```python
from build123d import *

# Parameters (mm, degrees)
F0_W     = 714.375
F0_H     = 603.123
F1_DEPTH = 3.175
F2_W     = 720.725
F2_H     = 609.473
F2_W_2   = 714.375
F2_H_2   = 603.123
F3_DEPTH = 28.575


with BuildPart() as f1:
    # F0 (on Top) → F1 (new body)
    with BuildSketch(Plane.XY):
        Rectangle(F0_W, F0_H)
    extrude(amount=F1_DEPTH)

    # F2 (on face) → F3 (join)
    with BuildSketch(Plane.XY.offset(3.175)):
        Rectangle(F2_W, F2_H)
        Rectangle(F2_W_2, F2_H_2, mode=Mode.SUBTRACT)
    extrude(amount=-F3_DEPTH)


solid = f1.part
```
Work out the finished part from the listing and answer in its coordinate system (mm). A direction names the side the tool comes from. Round coordinates to 2 decimals unless told otherwise and drop trailing zeros. Write each loop counter-clockwise with the first axis right and the second up, starting at its lowest first coordinate (ties: lowest second). Pieces come first, ordered by that corner, then holes.
1) A cutting plane is placed at A-A on z = -19.5. Determine the outline of the cut face in (x, y), and give its area (3 significant figures).
2) Consider probe 1 along X at (y, z) = (179.5, -22.25); probe 2 along Y at (x, z) = (149, -4); probe 3 along Z at (x, y) = (-126, -265.5) (3 decimals). Determine where each line is inside the solid, lowest interval first.
3) Which of the six approach directions +Z, -Z, +X, -X, +Y, -Y give full straight-line access (tool end or side, diameter ignored) to faces 1 (the face through (-5, -301.562, -13)), 2 (the face through (-5, -304.736, -11))?
4) Determine the mould class of faces 3 (the face through (360.362, -4, -11)), 4 (the face through (357.188, -4, -13)), 5 (the face through (-360.362, -4, -11)) for opening direction X: pulls with the +X half, pulls with the -X half, needs draft (parallel to the pull), parting line crosses it, or undercut.
5) A cutting plane is placed at B-B on x = 34.5. Determine the outline of the cut face in (y, z) (1 decimal).
6) A cutting plane is placed at C-C on y = -72. Determine the outline of the cut face in (x, z) (1 decimal), and give its area (3 significant figures).
Entries:
1. outline: (-360.36, -304.74) - (360.36, -304.74) - (360.36, 304.74) - (-360.36, 304.74) - close; hole (-357.19, -301.56) - (357.19, -301.56) - (357.19, 301.56) - (-357.19, 301.56) - close
1. area: 8,410 mm2
2. probe 1: x = -360.36 to -357.19, 357.19 to 360.36
2. probe 2: y = -304.74 to -301.56, 301.56 to 304.74
2. probe 3: z = 0 to 3.175
3. face 1: -Z
3. face 2: +Z, -Z, +X, -X, -Y
4. face 3: pulls with the +X half
4. face 4: undercut
4. face 5: pulls with the -X half
5. outline: (-304.7, -25.4) - (-301.6, -25.4) - (-301.6, 0) - (301.6, 0) - (301.6, -25.4) - (304.7, -25.4) - (304.7, 3.2) - (-304.7, 3.2) - close
6. outline: (-360.4, -25.4) - (-357.2, -25.4) - (-357.2, 0) - (357.2, 0) - (357.2, -25.4) - (360.4, -25.4) - (360.4, 3.2) - (-360.4, 3.2) - close
6. area: 2,450 mm2
